Design review of the part built by this model. Coordinates are the model's own, in mm. A direction names the side the tool comes from. Round coordinates to 2 decimals unless told otherwise and drop trailing zeros. Order: outer loops, then holes, each group sorted by start corner. A loop starts at its lowest first (then second) coordinate and runs counter-clockwise, first axis right, second up. Notation, with made-up numbers: (-12, 88.25) - (24, 88.25) arc R22 ccw to (24, 103.25) - close; hole circle Ø2 at (36.5, 34). An arc over 180 degrees is marked (long way). Write item = value, one per line.
from build123d import *

# Parameters (mm, degrees)
SKETCH023_R     = 10.7
SKETCH023_R_2   = 1.65
PAD002_DEPTH    = 4
SKETCH022_R     = 3
POCKET002_DEPTH = 2
CHAMFER002_SIZE = 0.4


with BuildPart() as part:
    # Sketch021 (on XZ_Plane004 of Origin012) → Revolution002 (revolve)
    with BuildSketch(Plane.XZ):
        with BuildLine():
            Line((11.25, 11), (10.85, 31))
            ThreePointArc((10.85, 31), (10.034163, 31.783843), (9.25032, 30.968006))
            Line((9.25032, 30.968006), (9.65032, 10.968006))
            ThreePointArc((9.65032, 10.968006), (9.704303, 10.111313), (9.831558, 9.262405))
            Line((10.549746, 5.562561), (9.831558, 9.262405))
            ThreePointArc((10.7, 4), (10.66235, 4.784884), (10.549746, 5.562561))
            Line((10.7, 4), (12.5, 4))
            ThreePointArc((12.5, 4), (12.419287, 5.267973), (12.178449, 6.515477))
            Line((12.178449, 6.515477), (11.518423, 9.054966))
            ThreePointArc((11.25, 11), (11.327186, 10.019613), (11.518423, 9.054966))
        make_face()
    revolve(axis=Axis((0, 0, 0), (0, 0, 1)))

    # Sketch023 (on Face1 of Revolution002) → Pad002 (new body)
    with BuildSketch(Plane(origin=(0, 0, 4), x_dir=(1, 0, 0), z_dir=(0, 0, -1))):
        with BuildLine():
            ThreePointArc((5.46875, 11.24023), (0, 12.5), (-5.46875, 11.24023))
            Line((-5.46875, 11.24023), (-18.40625, 4.945701))
            ThreePointArc((-18.40625, 4.945701), (-21.5, 0), (-18.40625, -4.945701))
            Line((-18.40625, -4.945701), (-5.46875, -11.24023))
            ThreePointArc((-5.46875, -11.24023), (0, -12.5), (5.46875, -11.24023))
            Line((5.46875, -11.24023), (18.40625, -4.945701))
            ThreePointArc((18.40625, -4.945701), (21.5, 0), (18.40625, 4.945701))
            Line((5.46875, 11.24023), (18.40625, 4.945701))
        make_face()
        Circle(SKETCH023_R, mode=Mode.SUBTRACT)
        with Locations((-16, 0)):
            Circle(SKETCH023_R_2, mode=Mode.SUBTRACT)
        with Locations((16, 0)):
            Circle(SKETCH023_R_2, mode=Mode.SUBTRACT)
    extrude(amount=PAD002_DEPTH)

    # Sketch022 (on Face3 of Pad002) → Pocket002 (cut)
    with BuildSketch(Plane.XY.offset(4)):
        with Locations((-16, 0)):
            Circle(SKETCH022_R)
        with Locations((16, 0)):
            Circle(SKETCH022_R)
    extrude(amount=-POCKET002_DEPTH, mode=Mode.SUBTRACT)

    # Chamfer002
    chamfer002_edges = [part.edges().sort_by_distance(p)[0] for p in [
        (-10.7, 0, 0),
        (-17.65, 0, 0),
        (14.35, 0, 0),
        (-11.9375, 8.092966, 0),
    ]]
    chamfer(chamfer002_edges, length=CHAMFER002_SIZE)


with BuildPart() as part_1:
    # Body005 placement: moved
    add(part.part.moved(Location((0, 30, 0))))


solid = part_1.part
Item 1: The part is to be moulded in two halves that separate along Y. For faces 1 (the face through (-11.847, 21.863, 2.225)), 2 (the face through (-15.11, 28.61, 1.21)), 3 (the face through (-2.395, 19.215, 21.14)), say which applies: +Y half, -Y half, draft (parallel to the pull), parting line (faces both ways), or undercut.
Data:
face_1 = -Y half
face_2 = undercut
face_3 = parting line
Item 2: Insertion check: P1, Ø5, axis at y = 32, z = 17, coming from the +X side; P2, Ø4, axis at x = 6, z = 23.5, coming from the +Y side; P3, Ø3, axis at x = 9, z = 13.5, coming from the -Y side. Each pin has a flat end and moves straight along its axis. Give the tip position at first contact, or say it passes through.
Data:
P1 = 11.16
P2 = 40.25
P3 = 21.68
Item 3: For faces 4 (the face through (-1.39, 19.39, 2.23)), 5 (the face through (-14.7, 28.7, 2)), 6 (the face through (-0.08, 42.21, 0.11)), list the 3-axis set-ups (+Z, -Z, +X, -X, +Y, -Y) from which the entire face can be reached by the end or side of a thin tool; tool diameter is ignored.
Data:
face_4 = -Z
face_5 = +Z
face_6 = -Z, +Y
Item 4: Take a section at A-A, the plane x = 16. State the section outline as (y, z) points.
Data:
outline = (23.88, 0.4) - (24.33, 0) - (27.95, 0) - (28.35, 0.4) - (28.35, 2) - (27, 2) - (27, 4) - (23.88, 4) - close; (31.65, 0.4) - (32.05, 0) - (35.67, 0) - (36.12, 0.4) - (36.12, 4) - (33, 4) - (33, 2) - (31.65, 2) - close
Item 5: Take a section at D-D, the plane z = 12.5. State the section outline as (x, y) points, and give its area (3 significant figures).
Data:
outline = circle Ø22.44 at (0, 30); hole circle Ø19.24 at (0, 30)
area = 105 mm2
Item 6: Take a section at C-C, the plane y = 29.5. Count the separate pieces of the cut face and the enclosed holes in it, and give its area (3 significant figures).
Data:
separate_pieces = 4
enclosed_holes = 0
area = 140 mm2
Item 7: Take a section at B-B, the plane z = 20.5. State the section outline as (x, y) points, and give its area (3 significant figures).
Data:
outline = circle Ø22.12 at (0, 30); hole circle Ø18.92 at (0, 30)
area = 103 mm2
Item 8: For line 1 along Y through (x, z) = (0, 1.95); line 2 along Y through (x, z) = (-1, 12.5); line 3 along Z through (x, y) = (11.5, 35.5), list the stretches that pass through material, from the lowest coordinate up. Write a range as [from, to].
Data:
line_1 = [17.5, 19.3], [40.7, 42.5]
line_2 = [18.82, 20.43], [39.57, 41.18]
line_3 = [0, 4]
